CAD build for the part. Positions are in the model's coordinates, mm. Face numbers are marked on the shaded views. A direction names the side the tool comes from. Coordinates: 2 decimals unless noted, no trailing zeros. Write each loop counter-clockwise with the first axis right and the second up, starting at its lowest first coordinate (ties: lowest second). Pieces come first, ordered by that corner, then holes. Notation, with made-up numbers: (88, -30) - (100, -30) arc R14 cw to (100, -8) - close; hole circle Ø10 at (61.25, -24.75). An arc over 180 degrees is marked (long way). Answer in a Markdown table with one row per item. Add a question column.
Q1. Band-saw the part on B-B (z = 4.75). List the corners of the cut face in (x, y), and give its area (3 significant figures).
Q2. 3-axis set-ups, long thin cutter, end or side, ignore diameter. For the marked faces 1 and 2: which of +Z, -Z, +X, -X, +Y, -Y reach the whole face in a straight line?
Q3. Pin check, flat tip, straight feed: pin 1 (15 mm diameter, centred on x = -4, y = 5.5, fed in from +Z). Stop position of the tip, or through.
Q4. Drill centre lines: line 1 along Y through (x, z) = (-1, 7.75); line 2 along X through (y, z) = (-11.5, 5.75); line 3 along X through (y, z) = (13.5, 1). Where is each one in solid material? Low to high. Write a range as from..to.
Q5. Band-saw the part on D-D (x = -1.5). List the corners of the cut face in (y, z).
Q6. Two-plate mould, pull along X, no slides. Class the marked faces 3, 4 and 5: +X half, -X half, draft (parallel to the pull), parting line (faces both ways), or undercut.
Q7. Band-saw the part on A-A (x = -14). List the corners of the cut face in (y, z).
Q8. Band-saw the part on C-C (y = -6.5). List the corners of the cut face in (x, z).
```python
from build123d import *

# Parameters (mm, degrees)
SKETCH2_W           = 54.5
SKETCH2_H           = 34.5
BOSS_EXTRUDE1_DEPTH = 8
SHELL1_T            = -2
FILLET2_R           = 4
SKETCH3_W           = 11
SKETCH3_H           = 11
CUT_EXTRUDE1_DEPTH  = 26


with BuildPart() as part:
    # Sketch2 → Boss-Extrude1 (new body)
    with BuildSketch(Plane.XY):
        Rectangle(SKETCH2_W, SKETCH2_H)
    extrude(amount=BOSS_EXTRUDE1_DEPTH)

    # Shell1
    shell1_openings = [part.faces().sort_by_distance(p)[0] for p in [
        (0, 0, 8),
    ]]
    offset(amount=SHELL1_T, openings=shell1_openings, kind=Kind.INTERSECTION)

    # Fillet2
    fillet2_edges = [part.edges().sort_by_distance(p)[0] for p in [
        (27.25, -17.25, 4),
        (-27.25, -17.25, 4),
        (-27.25, 17.25, 4),
        (27.25, 17.25, 4),
    ]]
    fillet(fillet2_edges, radius=FILLET2_R)

    # Sketch3 → Cut-Extrude1 (cut)
    with BuildSketch(Plane(origin=(0, 0, -10), x_dir=(-1, 0, 0), z_dir=(0, 0, -1))):
        with Locations((17.75, 8.75)):
            Rectangle(SKETCH3_W, SKETCH3_H)
    extrude(amount=-CUT_EXTRUDE1_DEPTH, mode=Mode.SUBTRACT)


solid = part.part
```
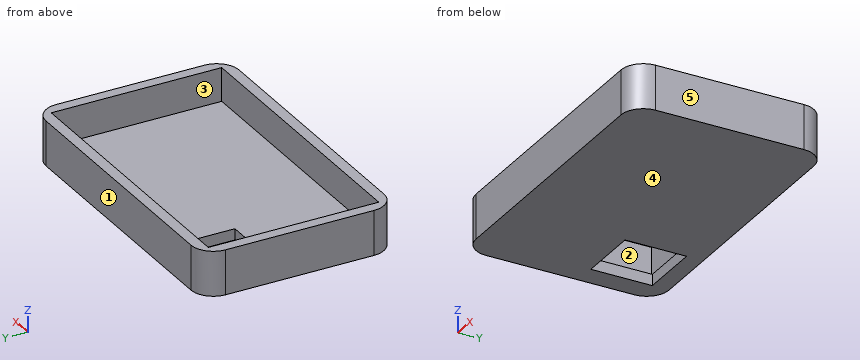
Checked values:
| question | item | result |
|---|---|---|
| 1 | outline | (-27.25, -13.25) arc R4 ccw to (-23.25, -17.25) - (23.25, -17.25) arc R4 ccw to (27.25, -13.25) - (27.25, 13.25) arc R4 ccw to (23.25, 17.25) - (-23.25, 17.25) arc R4 ccw to (-27.25, 13.25) - close; hole (-25.25, -15.25) - (25.25, -15.25) - (25.25, 15.25) - (-25.25, 15.25) - close |
| 1 | area | 326 mm² |
| 2 | face 1 | +Z, -Z, +X, -X, +Y |
| 2 | face 2 | +Z |
| 3 | pin 1 | stops at z = 2 |
| 4 | line 1 | y = -17.25..-15.25, 15.25..17.25 |
| 4 | line 2 | x = -27.25..-25.25, 25.25..27.25 |
| 4 | line 3 | x = -27.24..-23.25, -12.25..27.24 |
| 5 | outline | (-17.25, 0) - (17.25, 0) - (17.25, 8) - (15.25, 8) - (15.25, 2) - (-15.25, 2) - (-15.25, 8) - (-17.25, 8) - close |
| 6 | face 3 | undercut |
| 6 | face 4 | draft |
| 6 | face 5 | +X half |
| 7 | outline | (-17.25, 0) - (3.25, 0) - (3.25, 2) - (-15.25, 2) - (-15.25, 8) - (-17.25, 8) - close; (14.25, 0) - (17.25, 0) - (17.25, 8) - (15.25, 8) - (15.25, 2) - (14.25, 2) - close |
| 8 | outline | (-27.25, 0) - (27.25, 0) - (27.25, 8) - (25.25, 8) - (25.25, 2) - (-25.25, 2) - (-25.25, 8) - (-27.25, 8) - close |
